Can you work these out from the model? Positions are in its coordinate system, mm. Face numbers are marked on the shaded views. A direction names the side the tool comes from. Coordinates: 2 decimals unless noted, no trailing zeros. Order: outer loops, then holes, each group sorted by start corner. A loop starts at its lowest first (then second) coordinate and runs counter-clockwise, first axis right, second up. Notation, with made-up numbers: (56.25, -14.75) - (71.25, -14.75) arc R15 ccw to (71.25, 7.25) - close; hole circle Ø5 at (17.5, 3). An arc over 180 degrees is marked (long way). Return JSON: item names as keys, results as strings. Group by question number.
1) If I drill on line 1 along X through (y, z) = (60.75, -2.25); line 2 along Y through (x, z) = (0, -5.35), over which ranges is the centre line in solid material (lowest first)?
2) Which directions (+Z, -Z, +X, -X, +Y, -Y) give clear straight access to the entire face, cutting with the end or side of a thin tool? Please do the marked faces 1, 2, 3 and 4.
3) Imagine slicing it at B-B (y = 65). Write out the boundary of the cut face in (x, z).
4) Imagine slicing it at D-D (z = 0). Write out the boundary of the cut face in (x, y) (3 decimals), and give its area (3 significant figures).
5) For pin 1 Ø1.5 at (x, z) = (6, -5) entering from +Y; pin 2 Ø3 at (y, z) = (66, -2.5) entering from -X; pin 3 Ø5 at (x, y) = (-3, 67) entering from +Z; pin 4 Ø1 at (x, y) = (3.5, 64) entering from -Z, each with a flat end and sliding along its axis, tell me the tip position at first contact or that it passes through.
6) Imagine slicing it at A-A (x = 0). Write out the boundary of the cut face in (y, z) (3 decimals), and give its area (3 significant figures).
7) Imagine slicing it at C-C (y = 62). Write out the boundary of the cut face in (x, z).
8) If we mould it in two halves opening along Z, with no side actions, what happens to the marked faces 5, 6 and 7? For each: pulls with the +Z half, pulls with the -Z half, needs draft (parallel to the pull), parting line crosses it, or undercut.
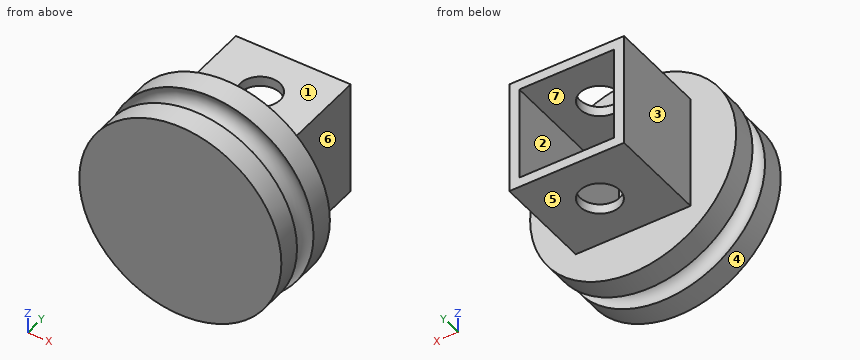
```python
from build123d import *

# Parameters (mm, degrees)
CYLINDER019_R     = 10.125
CYLINDER019_DEPTH = 7
BOX016_W          = 11.5
BOX016_H          = 11.5
BOX016_DEPTH      = 10
CYLINDER023_R     = 10.325
CYLINDER023_DEPTH = 2.5
BOX017_W          = 9.5
BOX017_H          = 9.5
BOX017_DEPTH      = 15
CYLINDER020_R     = 2
CYLINDER020_DEPTH = 11.5
TORUS_R           = 1.25


with BuildPart() as part:
    # Cylinder019 → Cylinder019 (join)
    with BuildSketch(Plane.XZ):
        Circle(CYLINDER019_R)
    extrude(amount=CYLINDER019_DEPTH)

    # Box016 → Box016 (join)
    with BuildSketch(Plane(origin=(-5.75, 0, 5.75), x_dir=(1, 0, 0), z_dir=(0, 1, 0))):
        with Locations((5.75, 5.75)):
            Rectangle(BOX016_W, BOX016_H)
    extrude(amount=BOX016_DEPTH)

    # Cylinder023 → Cylinder023 (join)
    with BuildSketch(Plane(origin=(0, 0, 0), x_dir=(-1, 0, 0), z_dir=(0, -1, 0))):
        Circle(CYLINDER023_R)
    extrude(amount=CYLINDER023_DEPTH)

    # Box017 → Box017 (cut)
    with BuildSketch(Plane(origin=(-4.75, 10, -4.75), x_dir=(1, 0, 0), z_dir=(0, -1, 0))):
        with Locations((4.75, 4.75)):
            Rectangle(BOX017_W, BOX017_H)
    extrude(amount=BOX017_DEPTH, mode=Mode.SUBTRACT)

    # Cylinder020 → Cylinder020 (cut)
    with BuildSketch(Plane(origin=(0, 5, 5.75), x_dir=(1, 0, 0), z_dir=(0, 0, -1))):
        Circle(CYLINDER020_R)
    extrude(amount=CYLINDER020_DEPTH, mode=Mode.SUBTRACT)

    # Torus → Torus (revolve, cut)
    with BuildSketch(Plane(origin=(0, -3.5, 0), x_dir=(1, 0, 0), z_dir=(0, 0, -1))):
        with Locations((9.625, 0)):
            Circle(TORUS_R)
    revolve(axis=Axis((0, -3.5, 0), (0, -1, 0)), mode=Mode.SUBTRACT)


with BuildPart() as part_1:
    # Body004 placement: moved
    add(part.part.moved(Location((0, 60, 0))))


solid = part_1.part
```
Calculated:
{
 "1": {"line 1": "-5.75 to -4.75, 4.75 to 5.75", "line 2": "53 to 63, 67 to 70"},
 "2": {"face 1": "+Z, +X, -X, +Y", "face 2": "+Y", "face 3": "+Z, -Z, -X, +Y", "face 4": "-Y"},
 "3": {"outline": "(-5.75, -5.75) - (-2, -5.75) - (-2, -4.75) - (-4.75, -4.75) - (-4.75, 4.75) - (-2, 4.75) - (-2, 5.75) - (-5.75, 5.75) - close; (2, -5.75) - (5.75, -5.75) - (5.75, 5.75) - (2, 5.75) - (2, 4.75) - (4.75, 4.75) - (4.75, -4.75) - (2, -4.75) - close"},
 "4": {"outline": "(-10.325, 57.536) arc R1.25 cw (long way) to (-10.125, 55.354) - (-10.125, 53) - (10.125, 53) - (10.125, 55.354) arc R1.25 cw (long way) to (10.325, 57.536) - (10.325, 60) - (5.75, 60) - (5.75, 70) - (4.75, 70) - (4.75, 55) - (-4.75, 55) - (-4.75, 70) - (-5.75, 70) - (-5.75, 60) - (-10.325, 60) - close", "area": "108 mm2"},
 "5": {"pin 1": "y = 70", "pin 2": "x = -5.75", "pin 3": "z = 5.75", "pin 4": "z = -5.75"},
 "6": {"outline": "(53, -10.125) - (55.354, -10.125) arc R1.25 cw (long way) to (57.536, -10.325) - (60, -10.325) - (60, -5.75) - (63, -5.75) - (63, -4.75) - (55, -4.75) - (55, 4.75) - (63, 4.75) - (63, 5.75) - (60, 5.75) - (60, 10.325) - (57.536, 10.325) arc R1.25 cw (long way) to (55.354, 10.125) - (53, 10.125) - close; (67, -5.75) - (70, -5.75) - (70, -4.75) - (67, -4.75) - close; (67, 4.75) - (70, 4.75) - (70, 5.75) - (67, 5.75) - close", "area": "99.9 mm2"},
 "7": {"outline": "(-5.75, -5.75) - (5.75, -5.75) - (5.75, 5.75) - (-5.75, 5.75) - close; hole (-4.75, -4.75) - (4.75, -4.75) - (4.75, 4.75) - (-4.75, 4.75) - close"},
 "8": {"face 5": "pulls with the -Z half", "face 6": "needs draft", "face 7": "undercut"}
}
